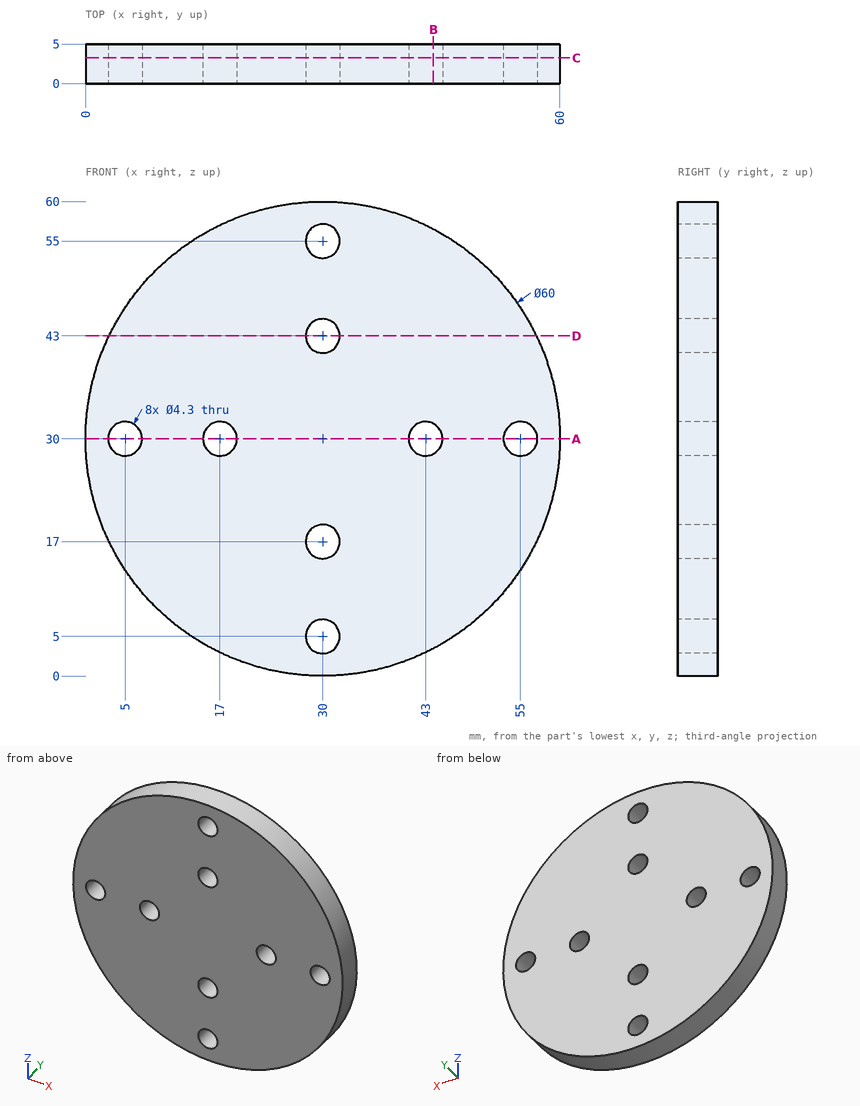
Can you work these out from the drawing? Everything is in mm from the part's minimum corner. Round coordinates to 2 decimals unless told otherwise and drop trailing zeros. Write each loop counter-clockwise with the first axis right and the second up, starting at its lowest first coordinate (ties: lowest second). Pieces come first, ordered by that corner, then holes. Notation, with made-up numbers: (23.25, 47) - (30.25, 47) arc R30 ccw to (30.25, 85) - close; hole circle Ø11 at (-7, 5.5). An arc over 180 degrees is marked (long way). Put each result on its own line as item: value. Start each with the question number.
(1) Will these pins go through, and if not, where does the flat tip stop? pin 1 (2.5 mm diameter, centred on x = 30, z = 17, fed in from +Y); pin 2 (1.5 mm diameter, centred on x = 45, y = 3, fed in from -Z); pin 3 (1.5 mm diameter, centred on x = 20, y = 1.5, fed in from +Z); pin 4 (3 mm diameter, centred on y = 2.5, z = 9.5, fed in from +X).
(2) I want a section at D-D, the plane z = 43. Please give me the cut outline in (x, y).
(3) I want a section at C-C, the plane y = 3.25. Give the number of separate pieces and of enclosed holes in the cut face, plus the area to 3 significant figures.
(4) I need wall thicknesses on probe 1 along X at (y, z) = (4.25, 30); probe 2 along X at (y, z) = (1.3, 55); probe 3 along Z at (x, y) = (18, 4.5). Which ranges of each line are inside material? Lowest first, please.
(5) I want a section at B-B, the plane x = 44. Please give me the cut outline in (y, z), plus the area to 3 significant figures.
(6) I want a section at A-A, the plane z = 30. Please give me the cut outline in (x, y), plus the area to 3 significant figures.
Here are the results:
1. pin 1: passes through
1. pin 2: stops at z = 3.6
1. pin 3: stops at z = 58.54
1. pin 4: stops at x = 53.22
2. outline: (2.96, 0) - (27.85, 0) - (27.85, 5) - (2.96, 5) - close; (32.15, 0) - (57.04, 0) - (57.04, 5) - (32.15, 5) - close
3. separate pieces: 1
3. enclosed holes: 8
3. area: 2,710 mm^2
4. probe 1: x = 0 to 2.85, 7.15 to 14.85, 19.15 to 40.85, 45.15 to 52.85, 57.15 to 60
4. probe 2: x = 13.42 to 27.85, 32.15 to 46.58
4. probe 3: z = 2.5 to 28.1, 31.9 to 57.5
5. outline: (0, 3.47) - (5, 3.47) - (5, 28.1) - (0, 28.1) - close; (0, 31.9) - (5, 31.9) - (5, 56.53) - (0, 56.53) - close
5. area: 246 mm^2
6. outline: (0, 0) - (2.85, 0) - (2.85, 5) - (0, 5) - close; (7.15, 0) - (14.85, 0) - (14.85, 5) - (7.15, 5) - close; (19.15, 0) - (40.85, 0) - (40.85, 5) - (19.15, 5) - close; (45.15, 0) - (52.85, 0) - (52.85, 5) - (45.15, 5) - close; (57.15, 0) - (60, 0) - (60, 5) - (57.15, 5) - close
6. area: 214 mm^2
